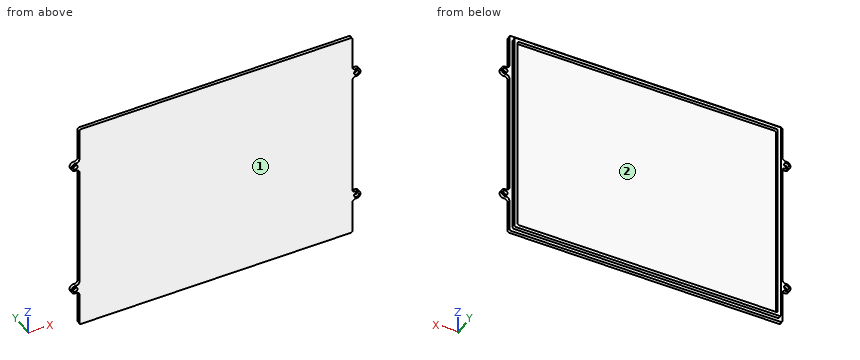
from build123d import *

# Parameters (mm, degrees)
EXTRUDE_1_DEPTH = 2
EXTRUDE_2_DEPTH = 2
SKETCH_3_R      = 1.45
EXTRUDE_5_DEPTH = 2


with BuildPart() as part:
    # 草图1 → 凸台-拉伸1 (new body)
    with BuildSketch(Plane(origin=(0, 0, 0), x_dir=(1, 0, 0), z_dir=(0, 1, 0))):
        with BuildLine():
            Line((-83.5, -67.25), (83.5, -67.25))
            ThreePointArc((83.5, -67.25), (84.207106781, -66.957106781), (84.5, -66.25))
            Line((84.5, -66.25), (84.5, 66.25))
            ThreePointArc((84.5, 66.25), (84.207106781, 66.957106781), (83.5, 67.25))
            Line((83.5, 67.25), (-83.5, 67.25))
            ThreePointArc((-83.5, 67.25), (-84.207106781, 66.957106781), (-84.5, 66.25))
            Line((-84.5, 66.25), (-84.5, -66.25))
            ThreePointArc((-84.5, -66.25), (-84.207106781, -66.957106781), (-83.5, -67.25))
        make_face()
    extrude(amount=EXTRUDE_1_DEPTH)

    # 草图2 → 凸台-拉伸2 (add)
    with BuildSketch(Plane(origin=(0, 2, 0), x_dir=(1, 0, 0), z_dir=(0, 1, 0))):
        with BuildLine():
            Line((-81.5, -65.25), (81.5, -65.25))
            ThreePointArc((81.5, -65.25), (82.207106781, -64.957106781), (82.5, -64.25))
            Line((82.5, -64.25), (82.5, 64.25))
            ThreePointArc((82.5, 64.25), (82.207106781, 64.957106781), (81.5, 65.25))
            Line((81.5, 65.25), (-81.5, 65.25))
            ThreePointArc((-81.5, 65.25), (-82.207106781, 64.957106781), (-82.5, 64.25))
            Line((-82.5, 64.25), (-82.5, -64.25))
            ThreePointArc((-82.5, -64.25), (-82.207106781, -64.957106781), (-81.5, -65.25))
        make_face()
        with BuildLine():
            Line((79.5, 63.25), (-79.5, 63.25))
            ThreePointArc((-79.5, 63.25), (-80.207106781, 62.957106781), (-80.5, 62.25))
            Line((-80.5, 62.25), (-80.5, -62.25))
            ThreePointArc((-80.5, -62.25), (-80.207106781, -62.957106781), (-79.5, -63.25))
            Line((-79.5, -63.25), (79.5, -63.25))
            ThreePointArc((79.5, -63.25), (80.207106781, -62.957106781), (80.5, -62.25))
            Line((80.5, -62.25), (80.5, 62.25))
            ThreePointArc((80.5, 62.25), (80.207106781, 62.957106781), (79.5, 63.25))
        make_face(mode=Mode.SUBTRACT)
    extrude(amount=EXTRUDE_2_DEPTH)

    # 草图3 → 凸台-拉伸5 (add)
    with BuildSketch(Plane.XZ):
        with BuildLine():
            Line((-84.5, 46.722135955), (-84.5, 37.777864045))
            ThreePointArc((-84.5, 37.777864045), (-85.166666667, 39.26857603), (-86.722222222, 39.765480025))
            ThreePointArc((-86.722222222, 39.765480025), (-89.5, 42.25), (-86.722222222, 44.734519975))
            ThreePointArc((-86.722222222, 44.734519975), (-85.166666667, 45.23142397), (-84.5, 46.722135955))
        make_face()
        with Locations((-87, 42.25)):
            Circle(SKETCH_3_R, mode=Mode.SUBTRACT)
        with BuildLine():
            Line((84.5, 46.722135955), (84.5, 37.777864045))
            ThreePointArc((84.5, 37.777864045), (85.166666667, 39.26857603), (86.722222222, 39.765480025))
            ThreePointArc((86.722222222, 39.765480025), (89.5, 42.25), (86.722222222, 44.734519975))
            ThreePointArc((86.722222222, 44.734519975), (85.166666667, 45.23142397), (84.5, 46.722135955))
        make_face()
        with Locations((87, 42.25)):
            Circle(SKETCH_3_R, mode=Mode.SUBTRACT)
        with BuildLine():
            Line((84.5, -46.722135955), (84.5, -37.777864045))
            ThreePointArc((84.5, -37.777864045), (85.166666667, -39.26857603), (86.722222222, -39.765480025))
            ThreePointArc((86.722222222, -39.765480025), (89.5, -42.25), (86.722222222, -44.734519975))
            ThreePointArc((86.722222222, -44.734519975), (85.166666667, -45.23142397), (84.5, -46.722135955))
        make_face()
        with Locations((87, -42.25)):
            Circle(SKETCH_3_R, mode=Mode.SUBTRACT)
        with BuildLine():
            Line((-84.5, -46.722135955), (-84.5, -37.777864045))
            ThreePointArc((-84.5, -37.777864045), (-85.166666667, -39.26857603), (-86.722222222, -39.765480025))
            ThreePointArc((-86.722222222, -39.765480025), (-89.5, -42.25), (-86.722222222, -44.734519975))
            ThreePointArc((-86.722222222, -44.734519975), (-85.166666667, -45.23142397), (-84.5, -46.722135955))
        make_face()
        with Locations((-87, -42.25)):
            Circle(SKETCH_3_R, mode=Mode.SUBTRACT)
    extrude(amount=-EXTRUDE_5_DEPTH)


solid = part.part
Work out the finished part from the listing and answer in its coordinate system (mm). Face numbers are marked on the shaded views. Coordinates: 2 decimals unless noted, no trailing zeros. Loops run counter-clockwise (first coordinate to the right, second up) from the corner with the lowest first, then second, coordinate; pieces in that order, holes last. Notation, with made-up numbers: (4.5, 56) -> (21.5, 56) arc R8 cw to (21.5, 70) -> close; hole circle Ø11 at (25.5, -6). An arc over 180 degrees is marked (long way). Write each question's results on one line, items separated by ' | '. Start each with the question number.
1) The mould has two halves that part along X. Classify the marked faces 1 and 2: pulls with the +X half, pulls with the -X half, needs draft (parallel to the pull), parting line crosses it, or undercut.
2) Find section B-B on z = 27. Determine the outline of the cut face in (x, y).
3) Find section C-C on x = -48.5. Determine the outline of the cut face in (y, z), then the cut area to 3 significant figures.
4) Find section A-A on y = 3. Determine the outline of the cut face in (x, z), then the cut area to 3 significant figures.
5) Flat-ended cylindrical pins translate along their axes: P1, Ø3.5, axis at x = -87, z = 42.25, coming from the -Y side; P2, Ø2, axis at y = 3.5, z = 23, coming from the -X side; P3, Ø0.6, axis at y = 0.5, z = 55, coming from the -X side; P4, Ø2, axis at x = -21, y = 3.5, coming from the +Z side. Find the tip coordinate at first contact, or state that the pin passes through.
6) Consider line 1 along Z through (x, y) = (87, 1.55); line 2 along Z through (x, y) = (-70, 3.65); line 3 along X through (y, z) = (2.45, -9). Determine where each line is inside the solid, lowest interval first.
Response values:
1) face 1: needs draft | face 2: undercut
2) outline: (-84.5, 0) -> (84.5, 0) -> (84.5, 2) -> (82.5, 2) -> (82.5, 4) -> (80.5, 4) -> (80.5, 2) -> (-80.5, 2) -> (-80.5, 4) -> (-82.5, 4) -> (-82.5, 2) -> (-84.5, 2) -> close
3) outline: (0, -67.25) -> (2, -67.25) -> (2, -65.25) -> (4, -65.25) -> (4, -63.25) -> (2, -63.25) -> (2, 63.25) -> (4, 63.25) -> (4, 65.25) -> (2, 65.25) -> (2, 67.25) -> (0, 67.25) -> close | area: 277 mm^2
4) outline: (-82.5, -64.25) arc R1 ccw to (-81.5, -65.25) -> (81.5, -65.25) arc R1 ccw to (82.5, -64.25) -> (82.5, 64.25) arc R1 ccw to (81.5, 65.25) -> (-81.5, 65.25) arc R1 ccw to (-82.5, 64.25) -> close; hole (-80.5, -62.25) arc R1 ccw to (-79.5, -63.25) -> (79.5, -63.25) arc R1 ccw to (80.5, -62.25) -> (80.5, 62.25) arc R1 ccw to (79.5, 63.25) -> (-79.5, 63.25) arc R1 ccw to (-80.5, 62.25) -> close | area: 1,170 mm^2
5) P1: stops at y = 0 | P2: stops at x = -82.5 | P3: stops at x = -84.5 | P4: stops at z = 65.25
6) line 1: z = -44.75 to -43.7, -40.8 to -39.75, 39.75 to 40.8, 43.7 to 44.75 | line 2: z = -65.25 to -63.25, 63.25 to 65.25 | line 3: x = -82.5 to -80.5, 80.5 to 82.5
